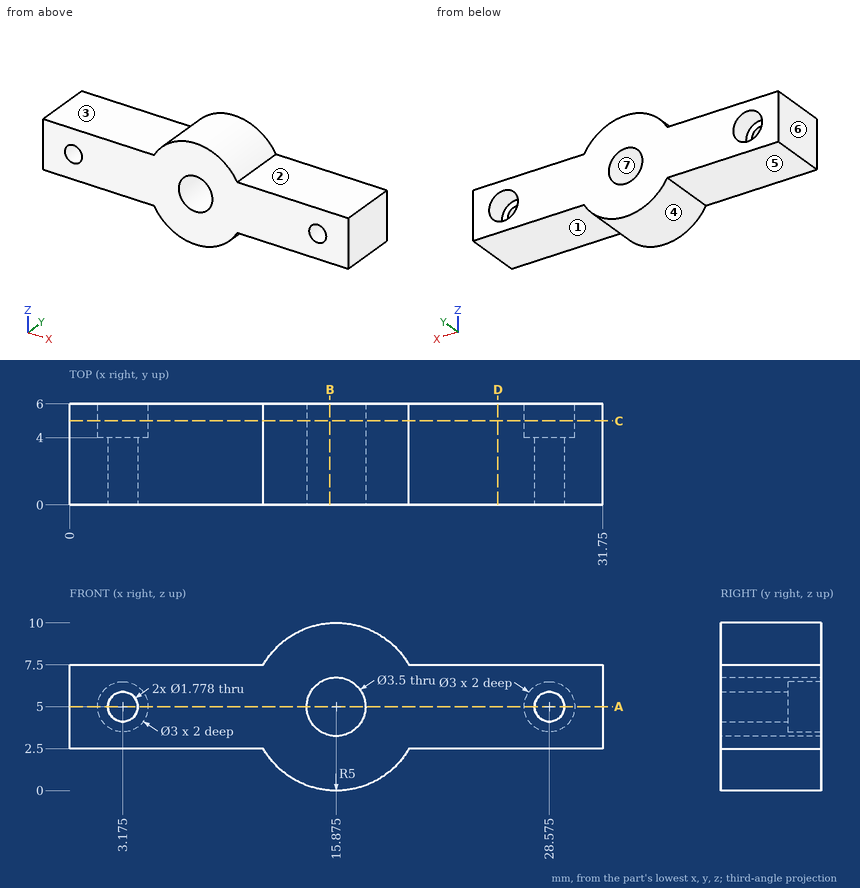
Job drawing, mm, ordinate dimensions from the low corner. One solid piece. A direction names the side the tool comes from. Give positions to 0.01 mm unless a question says otherwise; leave off trailing zeros. Loops run counter-clockwise (first coordinate to the right, second up) from the corner with the lowest first, then second, coordinate; pieces in that order, holes last. Notation, with made-up numbers: M 22,71.5 L 33,71.5 A9 cw 33,83.5 Z; hole C 83.5,84.5 d10. An arc over 180 degrees is marked long. Answer in a Markdown table with one row per item. Add a question column.
Item 1: Band-saw the part on C-C on y = 5. Give the cut face in (x, z) (3 decimals).
Item 2: Tool access for the marked faces 1, 2, 3 and 4: list every direction of +Z, -Z, +X, -X, +Y, -Y with a clear straight run to the whole face (end or side of a thin tool).
Item 3: Drop flat-ended pins along their axis: P1, Ø1.8, axis at x = 23, y = 4.5, coming from the +Z side; P2, Ø1.8, axis at x = 24.5, y = 3.5, coming from the -Z side; P3, Ø3, axis at x = 12.5, y = 3.5, coming from the -Z side. Give the stop position or say it passes through.
Item 4: Mould opens along Z. For the marked faces 5, 6 and 7 say: +Z half, -Z half, draft (parallel to the pull), parting line (faces both ways), or undercut.
Item 5: Band-saw the part on D-D on x = 25.5. Give the cut face in (y, z), then the cut area to 3 significant figures.
Item 6: Probe probe 1 along X at (y, z) = (2, 5) (3 decimals); probe 2 along X at (y, z) = (4.8, 5) (3 decimals); probe 3 along Z at (x, y) = (16, 3.5). List the from-to ranges inside material, lowest first.
Item 7: Band-saw the part on B-B on x = 15.5. Give the cut face in (y, z), then the cut area to 3 significant figures.
Item 8: Band-saw the part on A-A on z = 5. Give the cut face in (x, y) (3 decimals).
Reply:
| question | item | result |
|---|---|---|
| 1 | outline | M 0,2.5 L 11.545,2.5 A5 ccw 20.205,2.5 L 31.75,2.5 L 31.75,7.5 L 20.205,7.5 A5 ccw 11.545,7.5 L 0,7.5 Z; hole C 3.175,5 d3; hole C 15.875,5 d3.5; hole C 28.575,5 d3 |
| 2 | face 1 | -Z, +X, +Y, -Y |
| 2 | face 2 | +Z, +X, +Y, -Y |
| 2 | face 3 | +Z, -X, +Y, -Y |
| 2 | face 4 | -Z, +Y, -Y |
| 3 | P1 | stops at z = 7.5 |
| 3 | P2 | stops at z = 2.5 |
| 3 | P3 | stops at z = 0.36 |
| 4 | face 5 | -Z half |
| 4 | face 6 | draft |
| 4 | face 7 | undercut |
| 5 | outline | M 0,2.5 L 6,2.5 L 6,7.5 L 0,7.5 Z |
| 5 | area | 30.0 mm^2 |
| 6 | probe 1 | x = 0 to 2.286, 4.064 to 14.125, 17.625 to 27.686, 29.464 to 31.75 |
| 6 | probe 2 | x = 0 to 1.675, 4.675 to 14.125, 17.625 to 27.075, 30.075 to 31.75 |
| 6 | probe 3 | z = 0 to 3.25, 6.75 to 10 |
| 7 | outline | M 0,0.01 L 6,0.01 L 6,3.29 L 0,3.29 Z; M 0,6.71 L 6,6.71 L 6,9.99 L 0,9.99 Z |
| 7 | area | 39.3 mm^2 |
| 8 | outline | M 0,0 L 2.286,0 L 2.286,4 L 1.675,4 L 1.675,6 L 0,6 Z; M 4.064,0 L 14.125,0 L 14.125,6 L 4.675,6 L 4.675,4 L 4.064,4 Z; M 17.625,0 L 27.686,0 L 27.686,4 L 27.075,4 L 27.075,6 L 17.625,6 Z; M 29.464,0 L 31.75,0 L 31.75,6 L 30.075,6 L 30.075,4 L 29.464,4 Z |
